from build123d import *

# Parameters (mm, degrees)
F0_W     = 3.175
F0_H     = 3.175
F0_W_2   = 69.85
F0_H_2   = 12.7
F1_DEPTH = 3.175


with BuildPart() as f1:
    # F0 (on Front) → F1 (new body)
    with BuildSketch(Plane.XZ):
        Polygon((-67.174376142, 48.1953912664), (-79.874376142, 48.1953912664), (-79.874376142, 45.0203912664), (-79.874376142, 41.8453912664), (-79.874376142, 38.6703912664), (-79.874376142, 35.4953912664), (-67.174376142, 35.4953912664), align=None)
        with Locations((-81.461876142, 43.4328912664)):
            Rectangle(F0_W, F0_H)
        with Locations((-32.249376142, 41.8453912664)):
            Rectangle(F0_W_2, F0_H_2)
        with BuildLine():
            Line((15.375623858, 48.1953912664), (2.675623858, 48.1953912664))
            Line((2.675623858, 48.1953912664), (2.675623858, 35.4953912664))
            Line((2.675623858, 35.4953912664), (4.263123858, 35.4953912664))
            ThreePointArc((4.263123858, 35.4953912664), (6.3633054223, 39.4442476574), (10.811561358, 39.9103469283))
            ThreePointArc((10.811561358, 39.9103469283), (12.8969617645, 41.3416494053), (15.375623858, 41.8453912664))
            Line((15.375623858, 41.8453912664), (15.375623858, 48.1953912664))
        make_face()
        with BuildLine():
            Line((2.675623858, 35.4953912664), (-67.174376142, 35.4953912664))
            Line((-67.174376142, 35.4953912664), (-67.174376142, -2.6046087336))
            Line((-67.174376142, -2.6046087336), (28.075623858, -2.6046087336))
            Line((28.075623858, -2.6046087336), (28.075623858, 0.5703912664))
            Line((28.075623858, 0.5703912664), (28.075623858, 3.7453912664))
            Line((28.075623858, 3.7453912664), (28.075623858, 6.9203912664))
            Line((28.075623858, 6.9203912664), (28.075623858, 10.0953912664))
            Line((28.075623858, 10.0953912664), (28.075623858, 13.2703912664))
            Line((28.075623858, 13.2703912664), (28.075623858, 16.4453912664))
            Line((28.075623858, 16.4453912664), (28.075623858, 19.6203912664))
            Line((28.075623858, 19.6203912664), (28.075623858, 22.7953912664))
            Line((28.075623858, 22.7953912664), (28.075623858, 25.9703912664))
            Line((28.075623858, 25.9703912664), (28.075623858, 29.1453912664))
            Line((28.075623858, 29.1453912664), (28.075623858, 32.3203912664))
            Line((28.075623858, 32.3203912664), (28.075623858, 35.4953912664))
            Line((28.075623858, 35.4953912664), (21.725623858, 35.4953912664))
            ThreePointArc((21.725623858, 35.4953912664), (17.756873858, 29.6087837173), (10.811561358, 31.0804356046))
            ThreePointArc((10.811561358, 31.0804356046), (6.3633054223, 31.5465348754), (4.263123858, 35.4953912664))
            Line((4.263123858, 35.4953912664), (2.675623858, 35.4953912664))
        make_face()
        Polygon((-67.174376142, -2.6046087336), (-67.174376142, 35.4953912664), (-79.874376142, 35.4953912664), (-79.874376142, 32.3203912664), (-79.874376142, 29.1453912664), (-79.874376142, 25.9703912664), (-79.874376142, 22.7953912664), (-79.874376142, 19.6203912664), (-79.874376142, 16.4453912664), (-79.874376142, 13.2703912664), (-79.874376142, 10.0953912664), (-79.874376142, 6.9203912664), (-79.874376142, 3.7453912664), (-79.874376142, 0.5703912664), (-79.874376142, -2.6046087336), align=None)
        with Locations((-81.461876142, 37.0828912664)):
            Rectangle(F0_W, F0_H)
        with BuildLine():
            Line((28.075623858, 48.1953912664), (15.375623858, 48.1953912664))
            Line((15.375623858, 48.1953912664), (15.375623858, 41.8453912664))
            ThreePointArc((15.375623858, 41.8453912664), (19.8657519185, 39.985519327), (21.725623858, 35.4953912664))
            Line((21.725623858, 35.4953912664), (28.075623858, 35.4953912664))
            Line((28.075623858, 35.4953912664), (28.075623858, 38.6703912664))
            Line((28.075623858, 38.6703912664), (28.075623858, 41.8453912664))
            Line((28.075623858, 41.8453912664), (28.075623858, 45.0203912664))
            Line((28.075623858, 45.0203912664), (28.075623858, 48.1953912664))
        make_face()
        with Locations((-81.461876142, -1.0171087336)):
            Rectangle(F0_W, F0_H)
        with Locations((29.663123858, -1.0171087336)):
            Rectangle(F0_W, F0_H)
        with Locations((-81.461876142, 30.7328912664)):
            Rectangle(F0_W, F0_H)
        with Locations((29.663123858, 43.4328912664)):
            Rectangle(F0_W, F0_H)
        with Locations((29.663123858, 37.0828912664)):
            Rectangle(F0_W, F0_H)
        with Locations((-81.461876142, 5.3328912664)):
            Rectangle(F0_W, F0_H)
        with Locations((29.663123858, 5.3328912664)):
            Rectangle(F0_W, F0_H)
        with Locations((-81.461876142, 24.3828912664)):
            Rectangle(F0_W, F0_H)
        with Locations((29.663123858, 30.7328912664)):
            Rectangle(F0_W, F0_H)
        with Locations((-81.461876142, 11.6828912664)):
            Rectangle(F0_W, F0_H)
        with Locations((29.663123858, 11.6828912664)):
            Rectangle(F0_W, F0_H)
        with Locations((-81.461876142, 18.0328912664)):
            Rectangle(F0_W, F0_H)
        with Locations((29.663123858, 24.3828912664)):
            Rectangle(F0_W, F0_H)
        with Locations((29.663123858, 18.0328912664)):
            Rectangle(F0_W, F0_H)
    extrude(amount=F1_DEPTH)


solid = f1.part
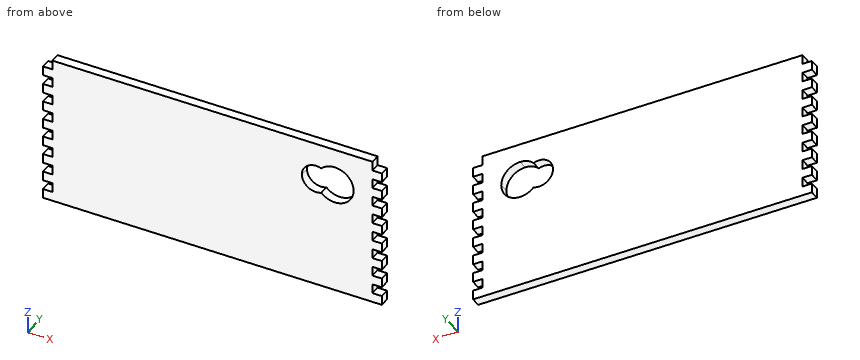
Verification items for the finished model (mm, model axes). Round coordinates to 2 decimals unless told otherwise and drop trailing zeros. Loops run counter-clockwise (first coordinate to the right, second up) from the corner with the lowest first, then second, coordinate; pieces in that order, holes last. Notation, with made-up numbers: (4, -14) - (19, -14) arc R20 cw to (19, 2) - close; hole circle Ø9 at (-21, 77). An arc over 180 degrees is marked (long way). Write item = value, one per line.
Q1. Depth check by flat-ended pin: pin 1 (1.6 mm diameter, centred on y = -2, z = 46.5, fed in from -X); pin 2 (1.6 mm diameter, centred on y = -1, z = 9, fed in from +X); pin 3 (3 mm diameter, centred on x = 6.5, z = 36, fed in from -Y). Enter the tip coordinate at first touch or a pass-through.
Here are the results:
pin_1 = -79.87
pin_2 = 28.08
pin_3 = through
Q2. Material ranges on L1, parallel to X at y = -1, z = 20; L2, parallel to X at y = -0.15, z = 32.5; L3, parallel to X at y = -2.95, z = 39.5, recorded low to high.
Here are the results:
L1 = -79.87 to 28.08
L2 = -79.87 to 5.32, 20.97 to 28.08
L3 = -79.87 to 6.45, 20.3 to 28.08
Q3. Sectioned sample at A-A on z = 21. Record the boundary of the cut face in (x, y) (3 decimals).
Here are the results:
outline = (-79.874, -3.175) - (28.076, -3.175) - (28.076, 0) - (-79.874, 0) - close
